Source: CAD feature listing. Evaluate the final solid. Frame: model axes, mm. Face numbers are marked on the shaded views. Round coordinates to 2 decimals unless told otherwise and drop trailing zeros. Loops run counter-clockwise (first coordinate to the right, second up) from the corner with the lowest first, then second, coordinate; pieces in that order, holes last. Notation, with made-up numbers: (-13, 44.25) -> (42, 44.25) arc R34 ccw to (42, 80.25) -> close; hole circle Ø10 at (-23, 25). An arc over 180 degrees is marked (long way). Put each result on its own line as item: value. Start each with the question number.
1. Material intervals for L1, parallel to Z at x = 15.5, y = 1.5; L2, parallel to Z at x = 0, y = 1.05, sorted ascending.
2. Cut plane C-C (y = 4.5). Return the cut outline in (x, z), then the cut area to 3 significant figures.
3. Cut plane A-A (x = 0). Return the cut outline in (y, z), then the cut area to 3 significant figures.
4. Contact query for flat-ended pins moving along their axis: pin 1 (3.5 mm diameter, centred on x = 16, z = 15, fed in from +Y); pin 2 (1.5 mm diameter, centred on x = -1, z = -7, fed in from +Y); pin 3 (10 mm diameter, centred on x = 3.5, y = 9.5, fed in from -Z). Output: stop coordinate, or through.
5. Cut plane B-B (z = 15.5). Return the cut outline in (x, y), then the cut area to 3 significant figures.
6. Draft query along Z for the marked faces 1, 2, 3 and 4. Return one class per face: pulls with the +Z half, pulls with the -Z half, needs draft (parallel to the pull), parting line crosses it, or undercut.
7. Cut plane D-D (x = 8.5). Return the cut outline in (y, z).
```python
from build123d import *

# Parameters (mm, degrees)
SKETCH_1_R           = 1.5
SKETCH_1_R_2         = 11
EXTRUDE_1_DEPTH      = 2
EXTRUDE_1_DEPTH_BACK = 60
EXTRUDE_2_DEPTH      = 22
SKETCH_2_R           = 11
SKETCH_2_R_2         = 1.5
EXTRUDE_3_DEPTH      = 60


with BuildPart() as part:
    # Sketch 1 → Extrude 1 (new body, two sides)
    with BuildSketch(Plane(origin=(0, 0, 0), x_dir=(1, 0, 0), z_dir=(0, 1, 0))) as extrude_1_sk:
        Polygon((-18.315463918, 21), (-21, 18.315463918), (-21, -18.402061856), (-18.402061856, -21), (18.402061856, -21), (21, -18.402061856), (21, 18.358762887), (18.358762887, 21), align=None)
        with Locations((-15.5, -15.5)):
            Circle(SKETCH_1_R, mode=Mode.SUBTRACT)
        with Locations((15.5, -15.5)):
            Circle(SKETCH_1_R, mode=Mode.SUBTRACT)
        Circle(SKETCH_1_R_2, mode=Mode.SUBTRACT)
        with Locations((-15.5, 15.5)):
            Circle(SKETCH_1_R, mode=Mode.SUBTRACT)
        with Locations((15.5, 15.5)):
            Circle(SKETCH_1_R, mode=Mode.SUBTRACT)
    extrude(amount=EXTRUDE_1_DEPTH)
    extrude(extrude_1_sk.sketch, amount=-EXTRUDE_1_DEPTH_BACK)



with BuildPart() as body_2:
    # Sketch 1_3 → Extrude 2 (new body)
    with BuildSketch(Plane(origin=(0, 0, 0), x_dir=(1, 0, 0), z_dir=(0, 1, 0))):
        with BuildLine():
            Line((1.870828693, 1.25), (-1.870828693, 1.25))
            ThreePointArc((-1.870828693, 1.25), (-0.65312152, -2.15312152), (2.25, 0))
            ThreePointArc((2.25, 0), (2.15312152, 0.65312152), (1.870828693, 1.25))
        make_face()
    extrude(amount=EXTRUDE_2_DEPTH)


with BuildPart() as part_1:
    add(part.part)

    add(body_2.part)  # Extrude 3 merges body 2
    # Sketch 2 → Extrude 3 (add)
    with BuildSketch(Plane.XZ.offset(60)):
        Circle(SKETCH_2_R)
        with Locations((-15.5, 15.5)):
            Circle(SKETCH_2_R_2)
        with Locations((15.5, 15.5)):
            Circle(SKETCH_2_R_2)
        with Locations((-15.5, -15.5)):
            Circle(SKETCH_2_R_2)
        with Locations((15.5, -15.5)):
            Circle(SKETCH_2_R_2)
    extrude(amount=-EXTRUDE_3_DEPTH)


solid = part_1.part
```
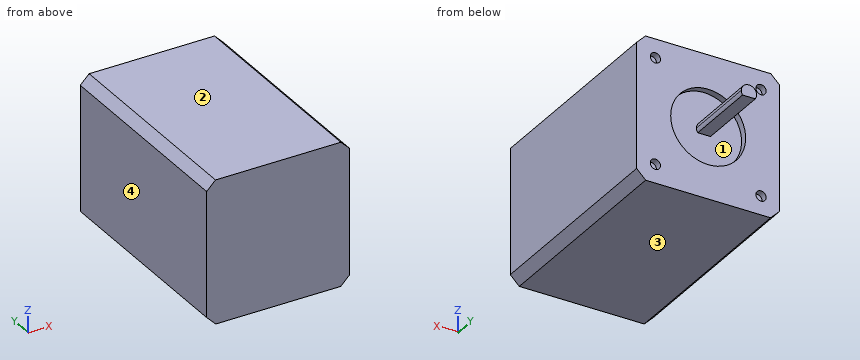
Solution:
1. L1: z = -21 to -17, -14 to 14, 17 to 21
1. L2: z = -21 to -11, -1.25 to 2.25, 11 to 21
2. outline: (-1.87, -1.25) -> (1.87, -1.25) arc R2.25 ccw (long way) to start
2. area: 13.3 mm^2
3. outline: (-60, -21) -> (2, -21) -> (2, -11) -> (0, -11) -> (0, -1.25) -> (22, -1.25) -> (22, 2.25) -> (0, 2.25) -> (0, 11) -> (2, 11) -> (2, 21) -> (-60, 21) -> close
3. area: 2,640 mm^2
4. pin 1: stops at y = 2
4. pin 2: stops at y = 0
4. pin 3: stops at z = -1.25
5. outline: (-21, -60) -> (21, -60) -> (21, 2) -> (17, 2) -> (17, 0) -> (14, 0) -> (14, 2) -> (-14, 2) -> (-14, 0) -> (-17, 0) -> (-17, 2) -> (-21, 2) -> close
5. area: 2,590 mm^2
6. face 1: undercut
6. face 2: pulls with the +Z half
6. face 3: pulls with the -Z half
6. face 4: needs draft
7. outline: (-60, -21) -> (2, -21) -> (2, -6.98) -> (0, -6.98) -> (0, 6.98) -> (2, 6.98) -> (2, 21) -> (-60, 21) -> close
